Job drawing, mm, ordinate dimensions from the low corner. One solid piece. A direction names the side the tool comes from. Coordinates: 2 decimals unless noted, no trailing zeros. Order: outer loops, then holes, each group sorted by start corner. A loop starts at its lowest first (then second) coordinate and runs counter-clockwise, first axis right, second up. Notation, with made-up numbers: (73.25, 59.5) - (97.25, 59.5) arc R21 ccw to (97.25, 74.5) - close; hole circle Ø7 at (-10.5, -21). An arc over 180 degrees is marked (long way). Use a Markdown table: item, result. Add a question column.
1) Saw through at C-C on x = 3.6. List the corners of the cut face in (y, z).
2) Saw through at A-A on y = 15. List the corners of the cut face in (x, z), then the cut area to 3 significant figures.
3) Saw through at B-B on z = 35. List the corners of the cut face in (x, y).
4) Drop flat-ended pins along their axis: P1, Ø6.5, axis at y = 15, z = 35, coming from the -X side; P2, Ø2.5, axis at x = 2, z = 37, coming from the +Y side. Give the stop position or say it passes through.
5) Wall check: L1, parallel to Y at x = 2.9, z = 35; L2, parallel to Y at x = 2, z = 48.5; L3, parallel to Y at x = 2.15, z = 36.5. Give the ranges that are in metal, low to high. Write a range as [from, to].
6) Tool access for the marked faces 1, 2 and 3: list every direction of +Z, -Z, +X, -X, +Y, -Y with a clear straight run to the whole face (end or side of a thin tool).
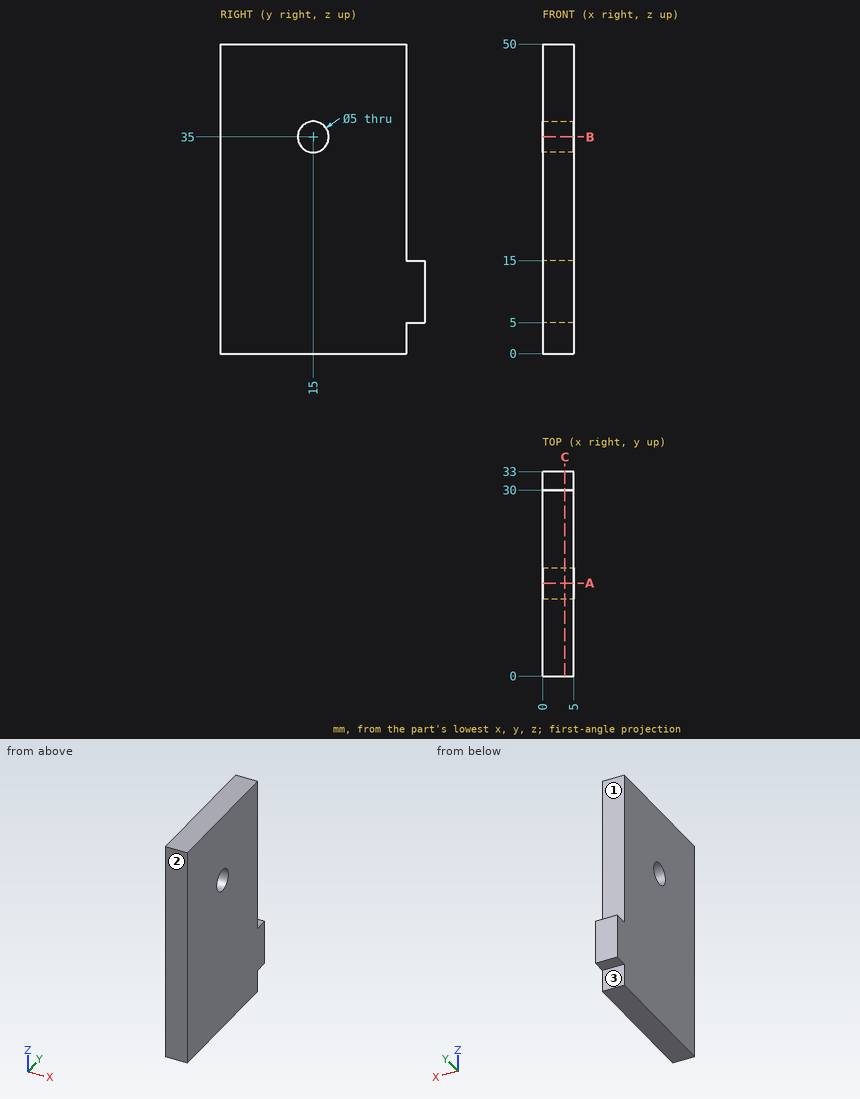
Results are:
| question | item | result |
|---|---|---|
| 1 | outline | (0, 0) - (30, 0) - (30, 5) - (33, 5) - (33, 15) - (30, 15) - (30, 50) - (0, 50) - close; hole circle Ø5 at (15, 35) |
| 2 | outline | (0, 0) - (5, 0) - (5, 32.5) - (0, 32.5) - close; (0, 37.5) - (5, 37.5) - (5, 50) - (0, 50) - close |
| 2 | area | 225 mm2 |
| 3 | outline | (0, 0) - (5, 0) - (5, 12.5) - (0, 12.5) - close; (0, 17.5) - (5, 17.5) - (5, 30) - (0, 30) - close |
| 4 | P1 | x = 0 |
| 4 | P2 | y = 30 |
| 5 | L1 | [0, 12.5], [17.5, 30] |
| 5 | L2 | [0, 30] |
| 5 | L3 | [0, 13], [17, 30] |
| 6 | face 1 | +Z, +X, -X, +Y |
| 6 | face 2 | +Z, -Z, +X, -X, -Y |
| 6 | face 3 | -Z, +X, -X, +Y |
